Source: CAD feature listing. Evaluate the final solid. Frame: model axes, mm. Face numbers are marked on the shaded views. A direction names the side the tool comes from. Give positions to 0.01 mm unless a question says otherwise; leave off trailing zeros. Order: outer loops, then holes, each group sorted by start corner. A loop starts at its lowest first (then second) coordinate and runs counter-clockwise, first axis right, second up.
1) Access query for the marked faces 1, 2, 3 and 4. Directions: +Z, -Z, +X, -X, +Y, -Y. A direction counts if a zero-diameter tool reaches every point of the face in a straight line with its end or side. Return the directions, or none.
2) Section A-A, the plane y = 117. Return loops of the section in (x, z), plus the area to 3 significant figures.
3) Section B-B, the plane z = 56. Return loops of the section in (x, y), plus the area to 4 significant figures.
4) Material intervals for line 1 (Z direction, x = 286.5, y = 62); line 2 (Z direction, x = -2.5, y = 188); line 3 (X direction, y = 172, z = -36), sorted ascending.
5) First-contact query: P1, Ø10, axis at y = 48.5, z = 51, coming from the +X side; P2, Ø3, axis at x = 347, y = 64, coming from the +Z side; P3, Ø4, axis at x = 195, y = 244, coming from the -Z side. Flat tips, straight axial feed; report the tip coordinate or a pass-through.
6) Section C-C, the plane x = -293. Return loops of the section in (y, z).
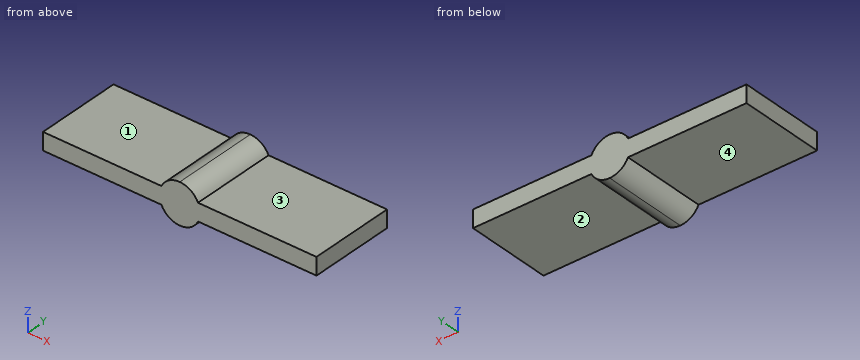
```python
from build123d import *

# Parameters (mm, degrees)
F1_DEPTH = 275


with BuildPart() as f1:
    # F0 (on Front) → F1 (new body)
    with BuildSketch(Plane.XZ):
        with BuildLine():
            ThreePointArc((-58.699841, -27.916459), (-63.405401, -14.309269), (-65, 0))
            ThreePointArc((-65, 0), (-63.405401, 14.309269), (-58.699841, 27.916459))
            Line((-58.699841, 27.916459), (-439.396739, 27.916459))
            Line((-439.396739, 27.916459), (-439.396739, -27.916459))
            Line((-439.396739, -27.916459), (-58.699841, -27.916459))
        make_face()
        with BuildLine():
            ThreePointArc((58.699841, 27.916459), (63.405401, 14.309269), (65, 0))
            ThreePointArc((65, 0), (63.405401, -14.309269), (58.699841, -27.916459))
            Line((58.699841, -27.916459), (439.396739, -27.916459))
            Line((439.396739, -27.916459), (439.396739, 27.916459))
            Line((439.396739, 27.916459), (58.699841, 27.916459))
        make_face()
        with BuildLine():
            Line((-65, 0), (0, 0))
            Line((0, 0), (0, 27.916459))
            Line((0, 27.916459), (-58.699841, 27.916459))
            ThreePointArc((-58.699841, 27.916459), (-63.405401, 14.309269), (-65, 0))
        make_face()
        with BuildLine():
            Line((0, 0), (65, 0))
            ThreePointArc((65, 0), (63.405401, 14.309269), (58.699841, 27.916459))
            Line((58.699841, 27.916459), (0, 27.916459))
            Line((0, 27.916459), (0, 0))
        make_face()
        with BuildLine():
            Line((0, 27.916459), (58.699841, 27.916459))
            ThreePointArc((58.699841, 27.916459), (34.716208, 54.95257), (0, 65))
            Line((0, 65), (0, 27.916459))
        make_face()
        with BuildLine():
            ThreePointArc((0, -65), (34.716208, -54.95257), (58.699841, -27.916459))
            Line((58.699841, -27.916459), (0, -27.916459))
            Line((0, -27.916459), (0, -65))
        make_face()
        with BuildLine():
            Line((0, -27.916459), (0, 0))
            Line((0, 0), (-65, 0))
            ThreePointArc((-65, 0), (-63.405401, -14.309269), (-58.699841, -27.916459))
            Line((-58.699841, -27.916459), (0, -27.916459))
        make_face()
        with BuildLine():
            ThreePointArc((58.699841, -27.916459), (63.405401, -14.309269), (65, 0))
            Line((65, 0), (0, 0))
            Line((0, 0), (0, -27.916459))
            Line((0, -27.916459), (58.699841, -27.916459))
        make_face()
        with BuildLine():
            ThreePointArc((-58.699841, -27.916459), (-34.716208, -54.95257), (0, -65))
            Line((0, -65), (0, -27.916459))
            Line((0, -27.916459), (-58.699841, -27.916459))
        make_face()
        with BuildLine():
            Line((0, 27.916459), (0, 65))
            ThreePointArc((0, 65), (-34.716208, 54.95257), (-58.699841, 27.916459))
            Line((-58.699841, 27.916459), (0, 27.916459))
        make_face()
    extrude(amount=-F1_DEPTH)


solid = f1.part
```
From the geometry:
1. face 1: +Z, -X, +Y, -Y
1. face 2: -Z, +X, +Y, -Y
1. face 3: +Z, +X, +Y, -Y
1. face 4: -Z, -X, +Y, -Y
2. outline: (-439.4, -27.92) - (-58.7, -27.92) arc R65 ccw to (0, -65) arc R65 ccw to (58.7, -27.92) - (439.4, -27.92) - (439.4, 27.92) - (58.7, 27.92) arc R65 ccw to (0, 65) arc R65 ccw to (-58.7, 27.92) - (-439.4, 27.92) - close
2. area: 55,300 mm2
3. outline: (-33, 0) - (33, 0) - (33, 275) - (-33, 275) - close
3. area: 18,150 mm2
4. line 1: z = -27.92 to 27.92
4. line 2: z = -64.95 to 64.95
4. line 3: x = -54.12 to 54.12
5. P1: stops at x = 45.92
5. P2: stops at z = 27.92
5. P3: stops at z = -27.92
6. outline: (0, -27.92) - (275, -27.92) - (275, 27.92) - (0, 27.92) - close
